from build123d import *

# Parameters (mm, degrees)
ESQUISSE1_R             = 20
BOSS_EXTRU_1_DEPTH      = 5
ENL_V_START             = -5
ENL_V_MAT_EXTRU_1_DEPTH = 5


with BuildPart() as part:
    # Esquisse1 → Boss.-Extru.1 (new body)
    with BuildSketch(Plane(origin=(0, 0, 0), x_dir=(1, 0, 0), z_dir=(0, 1, 0))):
        with Locations(Location((0, 0, 0), (0, 0, 270))):
            Circle(ESQUISSE1_R)
    extrude(amount=BOSS_EXTRU_1_DEPTH)

    # Esquisse2 → Enlèv. mat.-Extru.1 (cut)
    with BuildSketch(Plane(origin=(0, 5, 0), x_dir=(1, 0, 0), z_dir=(0, 1, 0)).offset(ENL_V_START)):
        with BuildLine():
            Line((-4.64704136, 15.319242341), (-3.90180644, 19.615705608))
            ThreePointArc((-3.90180644, 19.615705608), (-5.805693545, 19.138806715), (-7.653668647, 18.47759065))
            Line((-7.653668647, 18.47759065), (-4.64704136, 15.319242341))
        make_face()
        with BuildLine():
            Line((-1.569113842, 15.931480191), (0, 20))
            ThreePointArc((0, 20), (-1.960342807, 19.903694533), (-3.90180644, 19.615705608))
            Line((-3.90180644, 19.615705608), (-1.569113842, 15.931480191))
        make_face()
        with BuildLine():
            ThreePointArc((3.90180644, 19.615705608), (1.960342807, 19.903694533), (0, 20))
            Line((0, 20), (1.569113842, 15.931480191))
            Line((1.569113842, 15.931480191), (3.90180644, 19.615705608))
        make_face()
        with BuildLine():
            ThreePointArc((7.653668647, 18.47759065), (5.805693545, 19.138806715), (3.90180644, 19.615705608))
            Line((3.90180644, 19.615705608), (4.64704136, 15.319242341))
            Line((4.64704136, 15.319242341), (7.653668647, 18.47759065))
        make_face()
        with BuildLine():
            ThreePointArc((11.11140466, 16.629392246), (9.427934737, 17.638425287), (7.653668647, 18.47759065))
            Line((7.653668647, 18.47759065), (7.546385684, 14.1182946))
            Line((7.546385684, 14.1182946), (11.11140466, 16.629392246))
        make_face()
        with BuildLine():
            ThreePointArc((14.142135624, 14.142135624), (12.687865683, 15.460209067), (11.11140466, 16.629392246))
            Line((11.11140466, 16.629392246), (10.155726639, 12.374788715))
            Line((10.155726639, 12.374788715), (14.142135624, 14.142135624))
        make_face()
        with BuildLine():
            ThreePointArc((16.629392246, 11.11140466), (15.460209067, 12.687865683), (14.142135624, 14.142135624))
            Line((14.142135624, 14.142135624), (12.374788715, 10.155726639))
            Line((12.374788715, 10.155726639), (16.629392246, 11.11140466))
        make_face()
        with BuildLine():
            ThreePointArc((18.47759065, 7.653668647), (17.638425287, 9.427934737), (16.629392246, 11.11140466))
            Line((16.629392246, 11.11140466), (14.1182946, 7.546385684))
            Line((14.1182946, 7.546385684), (18.47759065, 7.653668647))
        make_face()
        with BuildLine():
            ThreePointArc((19.615705608, 3.90180644), (19.138806715, 5.805693545), (18.47759065, 7.653668647))
            Line((18.47759065, 7.653668647), (15.319242341, 4.64704136))
            Line((15.319242341, 4.64704136), (19.615705608, 3.90180644))
        make_face()
        with BuildLine():
            ThreePointArc((20, 0), (19.903694533, 1.960342807), (19.615705608, 3.90180644))
            Line((19.615705608, 3.90180644), (15.931480191, 1.569113842))
            Line((15.931480191, 1.569113842), (20, 0))
        make_face()
        with BuildLine():
            ThreePointArc((19.615705608, -3.90180644), (19.903694533, -1.960342807), (20, 0))
            Line((20, 0), (15.931480191, -1.569113842))
            Line((15.931480191, -1.569113842), (19.615705608, -3.90180644))
        make_face()
        with BuildLine():
            ThreePointArc((18.47759065, -7.653668647), (19.138806715, -5.805693545), (19.615705608, -3.90180644))
            Line((19.615705608, -3.90180644), (15.319242341, -4.64704136))
            Line((15.319242341, -4.64704136), (18.47759065, -7.653668647))
        make_face()
        with BuildLine():
            Line((-7.546385684, 14.1182946), (-7.653668647, 18.47759065))
            ThreePointArc((-7.653668647, 18.47759065), (-9.427934737, 17.638425287), (-11.11140466, 16.629392246))
            Line((-11.11140466, 16.629392246), (-7.546385684, 14.1182946))
        make_face()
        with BuildLine():
            Line((-10.155726639, 12.374788715), (-11.11140466, 16.629392246))
            ThreePointArc((-11.11140466, 16.629392246), (-12.687865683, 15.460209067), (-14.142135624, 14.142135624))
            Line((-14.142135624, 14.142135624), (-10.155726639, 12.374788715))
        make_face()
        with BuildLine():
            Line((-12.374788715, 10.155726639), (-14.142135624, 14.142135624))
            ThreePointArc((-14.142135624, 14.142135624), (-15.460209067, 12.687865683), (-16.629392246, 11.11140466))
            Line((-16.629392246, 11.11140466), (-12.374788715, 10.155726639))
        make_face()
        with BuildLine():
            Line((-14.1182946, 7.546385684), (-16.629392246, 11.11140466))
            ThreePointArc((-16.629392246, 11.11140466), (-17.638425287, 9.427934737), (-18.47759065, 7.653668647))
            Line((-18.47759065, 7.653668647), (-14.1182946, 7.546385684))
        make_face()
        with BuildLine():
            Line((-15.319242341, 4.64704136), (-18.47759065, 7.653668647))
            ThreePointArc((-18.47759065, 7.653668647), (-19.138806715, 5.805693545), (-19.615705608, 3.90180644))
            Line((-19.615705608, 3.90180644), (-15.319242341, 4.64704136))
        make_face()
        with BuildLine():
            Line((-15.931480191, 1.569113842), (-19.615705608, 3.90180644))
            ThreePointArc((-19.615705608, 3.90180644), (-19.903694533, 1.960342807), (-20, 0))
            Line((-20, 0), (-15.931480191, 1.569113842))
        make_face()
        with BuildLine():
            Line((-15.931480191, -1.569113842), (-20, 0))
            ThreePointArc((-20, 0), (-19.903694533, -1.960342807), (-19.615705608, -3.90180644))
            Line((-19.615705608, -3.90180644), (-15.931480191, -1.569113842))
        make_face()
        with BuildLine():
            Line((-15.319242341, -4.64704136), (-19.615705608, -3.90180644))
            ThreePointArc((-19.615705608, -3.90180644), (-19.138806715, -5.805693545), (-18.47759065, -7.653668647))
            Line((-18.47759065, -7.653668647), (-15.319242341, -4.64704136))
        make_face()
        with BuildLine():
            Line((-14.1182946, -7.546385684), (-18.47759065, -7.653668647))
            ThreePointArc((-18.47759065, -7.653668647), (-17.638425287, -9.427934737), (-16.629392246, -11.11140466))
            Line((-16.629392246, -11.11140466), (-14.1182946, -7.546385684))
        make_face()
        with BuildLine():
            Line((-12.374788715, -10.155726639), (-16.629392246, -11.11140466))
            ThreePointArc((-16.629392246, -11.11140466), (-15.460209067, -12.687865683), (-14.142135624, -14.142135624))
            Line((-14.142135624, -14.142135624), (-12.374788715, -10.155726639))
        make_face()
        with BuildLine():
            Line((-10.155726639, -12.374788715), (-14.142135624, -14.142135624))
            ThreePointArc((-14.142135624, -14.142135624), (-12.687865683, -15.460209067), (-11.11140466, -16.629392246))
            Line((-11.11140466, -16.629392246), (-10.155726639, -12.374788715))
        make_face()
        with BuildLine():
            Line((-7.546385684, -14.1182946), (-11.11140466, -16.629392246))
            ThreePointArc((-11.11140466, -16.629392246), (-9.427934737, -17.638425287), (-7.653668647, -18.47759065))
            Line((-7.653668647, -18.47759065), (-7.546385684, -14.1182946))
        make_face()
        with BuildLine():
            Line((-4.64704136, -15.319242341), (-7.653668647, -18.47759065))
            ThreePointArc((-7.653668647, -18.47759065), (-5.805693545, -19.138806715), (-3.90180644, -19.615705608))
            Line((-3.90180644, -19.615705608), (-4.64704136, -15.319242341))
        make_face()
        with BuildLine():
            Line((-1.569113842, -15.931480191), (-3.90180644, -19.615705608))
            ThreePointArc((-3.90180644, -19.615705608), (-1.960342807, -19.903694533), (0, -20))
            Line((0, -20), (-1.569113842, -15.931480191))
        make_face()
        with BuildLine():
            ThreePointArc((0, -20), (1.960342807, -19.903694533), (3.90180644, -19.615705608))
            Line((3.90180644, -19.615705608), (1.569113842, -15.931480191))
            Line((1.569113842, -15.931480191), (0, -20))
        make_face()
        with BuildLine():
            ThreePointArc((3.90180644, -19.615705608), (5.805693545, -19.138806715), (7.653668647, -18.47759065))
            Line((7.653668647, -18.47759065), (4.64704136, -15.319242341))
            Line((4.64704136, -15.319242341), (3.90180644, -19.615705608))
        make_face()
        with BuildLine():
            ThreePointArc((7.653668647, -18.47759065), (9.427934737, -17.638425287), (11.11140466, -16.629392246))
            Line((11.11140466, -16.629392246), (7.546385684, -14.1182946))
            Line((7.546385684, -14.1182946), (7.653668647, -18.47759065))
        make_face()
        with BuildLine():
            ThreePointArc((11.11140466, -16.629392246), (12.687865683, -15.460209067), (14.142135624, -14.142135624))
            Line((14.142135624, -14.142135624), (10.155726639, -12.374788715))
            Line((10.155726639, -12.374788715), (11.11140466, -16.629392246))
        make_face()
        with BuildLine():
            ThreePointArc((14.142135624, -14.142135624), (15.460209067, -12.687865683), (16.629392246, -11.11140466))
            Line((16.629392246, -11.11140466), (12.374788715, -10.155726639))
            Line((12.374788715, -10.155726639), (14.142135624, -14.142135624))
        make_face()
        with BuildLine():
            ThreePointArc((16.629392246, -11.11140466), (17.638425287, -9.427934737), (18.47759065, -7.653668647))
            Line((18.47759065, -7.653668647), (14.1182946, -7.546385684))
            Line((14.1182946, -7.546385684), (16.629392246, -11.11140466))
        make_face()
    extrude(amount=ENL_V_MAT_EXTRU_1_DEPTH, mode=Mode.SUBTRACT)


solid = part.part
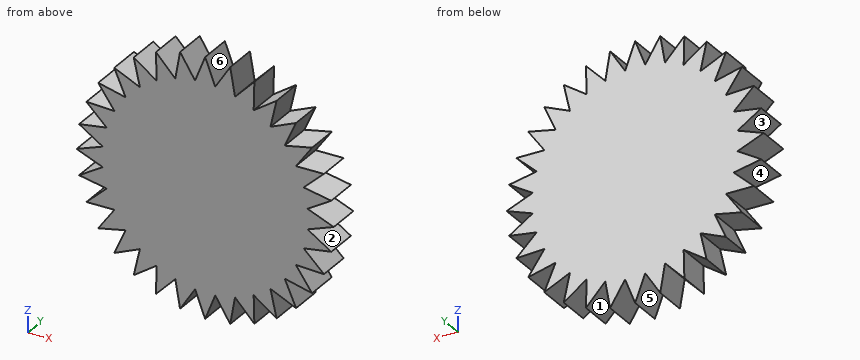
Work out the finished part from the listing and answer in its coordinate system (mm). Face numbers are marked on the shaded views. A direction names the side the tool comes from. Round coordinates to 2 decimals unless told otherwise and drop trailing zeros. Write each loop counter-clockwise with the first axis right and the second up, starting at its lowest first coordinate (ties: lowest second). Pieces come first, ordered by that corner, then holes.
1) A tool of negligible diameter and unlimited length cuts with its end or side. For the marked faces 4, 5 and 6, from which of +Z, -Z, +X, -X, +Y, -Y can it reach the whole face along a straight path? Write none if from no direction.
2) The mould has two halves that part along X. Classify the marked faces 1, 2 and 3: pulls with the +X half, pulls with the -X half, needs draft (parallel to the pull), parting line crosses it, or undercut.
3) A cutting plane is placed at B-B (x = 5.5). Give the vertices of the cut face in (y, z).
4) Given pin 1 Ø8 at (x, z) = (-13.5, 12) entering from +Y; pin 2 Ø1 at (x, y) = (12, 3) entering from -Z; pin 3 Ø1 at (x, y) = (10, 3) entering from +Z, each flat-ended and moving along its own axis, determine where each tip first touches the part or whether it passes through.
5) Straight lines are drawn through the part: line 1 (X direction, y = 2.65, z = 15); line 2 (Z direction, x = -14.5, y = 4.25); line 3 (Z direction, x = 18, y = 4.25). For each, find the intervals that lie inside material, in ascending order.
6) A cutting plane is placed at A-A (z = 3). Give the vertices of the cut face in (x, y), plus the area to 3 significant figures.
Completed:
1. face 4: -X, +Y, -Y
1. face 5: -Z, +Y, -Y
1. face 6: +Z, +Y, -Y
2. face 1: undercut
2. face 2: pulls with the +X half
2. face 3: pulls with the -X half
3. outline: (0, -16.22) - (5, -16.22) - (5, 16.22) - (0, 16.22) - close
4. pin 1: stops at y = 5
4. pin 2: stops at z = -13.41
4. pin 3: stops at z = 16.2
5. line 1: x = -10.75 to -8.8, -7.57 to 7.57, 8.8 to 10.75
5. line 2: z = -10.63 to -8.09, -7.56 to 7.56, 8.09 to 10.63
5. line 3: z = -7.64 to -7.2, -4.18 to -2.88, -0.77 to 0.77, 2.88 to 4.18, 7.2 to 7.64
6. outline: (-18.19, 0) - (18.19, 0) - (18.19, 5) - (-18.19, 5) - close
6. area: 182 mm2
